from build123d import *

# Parameters (mm, degrees)
F0_R     = 11.9016009371
F1_DEPTH = 5.08
F3_DEPTH = 5.08
F4_COUNT = 24
F4_ANGLE = 345


with BuildPart() as f1:
    # F0 (on Top) → F1 (new body)
    with BuildSketch(Plane.XY):
        Circle(F0_R)
        with BuildLine():
            ThreePointArc((-3.0120209, -0.8762828927), (0, 3.1369), (3.0120209, -0.8762828927))
            Line((3.0120209, -0.8762828927), (-3.0120209, -0.8762828927))
        make_face(mode=Mode.SUBTRACT)
    extrude(amount=F1_DEPTH)

    # F2 (on face) → F3 (cut, through all)
    with BuildSketch(Plane.XY.offset(5.08)):
        with BuildLine():
            ThreePointArc((-0.272684092, 9.968449005), (-0.1629528148, 9.8385506215), (0, 9.7899612874))
            Line((0, 9.7899612874), (0, 11.9016009371))
            ThreePointArc((0, 11.9016009371), (-0.5479117768, 11.8889821916), (-1.0946616999, 11.8511527131))
            Line((-1.0946616999, 11.8511527131), (-0.272684092, 9.968449005))
        make_face()
        with BuildLine():
            Line((0, 11.9016009371), (0, 9.7899612874))
            ThreePointArc((0, 9.7899612874), (0.1629528148, 9.8385506215), (0.272684092, 9.968449005))
            Line((0.272684092, 9.968449005), (1.0946616999, 11.8511527131))
            ThreePointArc((1.0946616999, 11.8511527131), (0.5479117768, 11.8889821916), (0, 11.9016009371))
        make_face()
    f3 = extrude(amount=-F3_DEPTH, mode=Mode.SUBTRACT)

    # F4: F3 ×24 about axis
    f4_axis = Axis((0, 0, 0), (0, 0, -1))
    for i in range(1, F4_COUNT):
        add(f3.rotate(f4_axis, i * F4_ANGLE / (F4_COUNT - 1)), mode=Mode.SUBTRACT)


solid = f1.part
Can you work these out from the model? Positions are in its coordinate system, mm. A direction names the side the tool comes from. Give positions to 0.01 mm unless a question says otherwise; leave off trailing zeros. Loops run counter-clockwise (first coordinate to the right, second up) from the corner with the lowest first, then second, coordinate; pieces in that order, holes last. Notation, with made-up numbers: (-22, 24) -> (22, 24) arc R15 cw to (22, 31) -> close; hole circle Ø1 at (52.25, -18.75). An arc over 180 degrees is marked (long way). Return JSON: item names as keys, results as strings.
Q1. I need wall thicknesses on probe 1 along X at (y, z) = (-8.5, 2.2) (3 decimals); probe 2 along X at (y, z) = (10, 3.45); probe 3 along Y at (x, z) = (-10.5, 2.5). Which ranges of each line are inside material? Lowest first, please.
Checks:
{"probe 1": "x = -7.349 to -5.225, -4.863 to 4.863, 5.225 to 7.349", "probe 2": "x = -4.89 to -3.2, -2.27 to -0.29, 0.29 to 2.27, 3.2 to 4.89", "probe 3": "y = -4.94 to -3.59, -2.2 to -0.5, 0.5 to 2.2, 3.59 to 4.94"}
Q2. We'd pull the mould along X, two halves only. Please class faces 5 (the face through (9.1, -6.04, 2.58)), 6 (the face through (-10.701, -2.165, 2.576)), 7 (the face through (6.059, -9.115, 2.576)), 8 (the face through (8.211, -7.236, 2.576)): released by +X, released by -X, zero draft, split by the parting line, or undercut.
Checks:
{"face 5": "released by +X", "face 6": "released by -X", "face 7": "undercut", "face 8": "undercut"}
Q3. For pin 1 Ø1 at (y, z) = (-3, 3) entering from -X; pin 2 Ø12 at (x, y) = (-5, -7.5) entering from -Z; pin 3 Ø1.5 at (y, z) = (-4, 4) entering from +X; pin 4 Ø2 at (y, z) = (-8, 2) entering from +X, each with a flat end and sliding along its axis, tell me the tip position at first contact or that it passes through.
Checks:
{"pin 1": "stops at x = -10.38", "pin 2": "stops at z = 0", "pin 3": "stops at x = 11.16", "pin 4": "stops at x = 9.63"}
Q4. I want a section at A-A, the plane x = -3.5. List the corners of the cut face in (y, z) for me, then the cut area to 3 significant figures.
Checks:
{"outline": "(-10.38, 0) -> (10.38, 0) -> (10.38, 5.08) -> (-10.38, 5.08) -> close", "area": "105 mm2"}
Q5. I want a section at B-B, the plane y = -6.25. List the corners of the cut face in (x, z) for me, then the cut area to 3 significant figures.
Checks:
{"outline": "(-9.26, 0) -> (9.26, 0) -> (9.26, 5.08) -> (-9.26, 5.08) -> close", "area": "94.0 mm2"}
Q6. On a 3-axis mill with a long thin cutter (end or side, diameter ignored), from which of +Z, -Z, +X, -X, +Y, -Y can I reach the whole of each face in a straight line? I mean faces 1 (the face through (-10.92, -0.69, 2.58)), 2 (the face through (-3.475, -10.35, 2.576)), 3 (the face through (10.9, -0.68, 2.58)), 4 (the face through (8.184, 7.226, 2.576)). Say none if no direction works.
Checks:
{"face 1": "+Z, -Z, -X", "face 2": "+Z, -Z, -Y", "face 3": "+Z, -Z, +X", "face 4": "+Z, -Z"}
